For this review, take the finished solid that the model builds, in its own axes (mm). A direction names the side the tool comes from. Round coordinates to 2 decimals unless told otherwise and drop trailing zeros. Write each loop counter-clockwise with the first axis right and the second up, starting at its lowest first coordinate (ties: lowest second). Pieces come first, ordered by that corner, then holes. Notation, with made-up numbers: M 88.5,42 L 116.5,42 A13 ccw 116.5,67 Z; hole C 1,55.25 d10. An arc over 180 degrees is marked long. Use one line per item in the form item = value. Start each with the question number.
Item 1: Add section B-B (x = -4.5). State the section outline as (y, z) points.
Item 2: Add section C-C (y = 4.7). State the section outline as (x, z) points, and give its area (3 significant figures).
Item 3: For faces 1 (the flat face through (62.7, 3, -0.6)), 2 (the flat face through (19.94, 2.96, 59.46)), 3 (the flat face through (-40.765, 2.958, 53.771)), 4 (the flat face through (18.81, 2.96, -59.82)), list the 3-axis set-ups (+Z, -Z, +X, -X, +Y, -Y) from which the entire face can be reached by the end or side of a thin tool; tool diameter is ignored.
Item 4: For line 1 (X direction, y = 1.2, z = 0); line 2 (X direction, y = 1.3, z = -24); line 3 (Z direction, x = -42.5, y = 4.3), list the stretches that pass through material, from the lowest coordinate up. Write a range as [from, to].
Item 5: Add section A-A (z = -30). State the section outline as (x, y) points.
Item 6: Draft analysis for pull direction X (two halves, no side actions). For faces 5 (the cylindrical face through (-17.345, 2.958, 68.973)), 6 (the flat face through (64.59, 2.96, -19.54)), 7 (the cylindrical face through (54.57, 2.96, -45.61)), state which applies: released by +X, released by -X, zero draft, split by the parting line, or undercut.
Item 7: For P1, Ø3, axis at x = 5, y = 5, coming from the -Z side; P2, Ø1, axis at x = -9, y = 1, coming from the -Z side, all flat-tipped, find the tip position at first contact; note any pin that passes through.
Item 8: Add section D-D (z = 0). State the section outline as (x, y) points.
from build123d import *

# Parameters (mm, degrees)
SKETCH1_R           = 3.3
SKETCH1_R_2         = 50.8
BOSS_EXTRUDE1_DEPTH = 6


with BuildPart() as part:
    # Sketch1 → Boss-Extrude1 (new body)
    with BuildSketch(Plane(origin=(0, 0, 0), x_dir=(1, 0, 0), z_dir=(0, 1, 0))):
        with BuildLine():
            ThreePointArc((-50.084292244, 23.446975703), (-54.118923856, 17.647036419), (-60.96, 19.41260294))
            Line((-60.96, 19.41260294), (-66.591321273, 24.972992034))
            ThreePointArc((-66.591321273, 24.972992034), (-70.926140308, -5.247572863), (-62.191041695, -34.501141038))
            Line((-62.191041695, -34.501141038), (-38.242542673, -40.255931215))
            ThreePointArc((-38.242542673, -40.255931215), (-34.829443057, -42.441548483), (-33.501782647, -46.270842108))
            ThreePointArc((-33.501782647, -46.270842108), (-34.53819598, -49.698469864), (-37.300158502, -51.97758102))
            Line((-37.300158502, -51.97758102), (-44.328576757, -55.615031086))
            ThreePointArc((-44.328576757, -55.615031086), (-16.926644335, -69.07635711), (13.594446222, -69.808634365))
            Line((13.594446222, -69.808634365), (26.468070107, -48.810586278))
            ThreePointArc((26.468070107, -48.810586278), (33.175934652, -46.026293541), (37.90723426, -51.536514664))
            Line((37.90723426, -51.536514664), (39.194754164, -59.344971531))
            ThreePointArc((39.194754164, -59.344971531), (60.464898794, -37.44396365), (70.592871518, -8.642967708))
            Line((70.592871518, -8.642967708), (54.600709616, 10.089329884))
            ThreePointArc((54.600709616, 10.089329884), (54.025534005, 17.329281943), (60.728117694, 20.126263296))
            Line((60.728117694, 20.126263296), (68.552267011, 18.937821619))
            ThreePointArc((68.552267011, 18.937821619), (54.296006916, 45.9347149), (30.03434774, 64.466986558))
            Line((30.03434774, 64.466986558), (7.277024245, 55.04613507))
            ThreePointArc((7.277024245, 55.04613507), (0.213681623, 56.736378783), (-0.375193452, 63.975229447))
            Line((-0.375193452, 63.975229447), (3.172876855, 71.049188964))
            ThreePointArc((3.172876855, 71.049188964), (-26.908121067, 65.833178722), (-52.030623785, 48.485756553))
            Line((-52.030623785, 48.485756553), (-50.103261295, 23.931052539))
            ThreePointArc((-50.103261295, 23.931052539), (-50.089036326, 23.68919988), (-50.084292244, 23.446975703))
        make_face()
        with Locations(Location((-18.837675977, -57.976405233, 0), (0, 0, 270))):
            Circle(SKETCH1_R, mode=Mode.SUBTRACT)
        with Locations(Location((-60.96, 0, 0), (0, 0, 270))):
            Circle(SKETCH1_R, mode=Mode.SUBTRACT)
        with Locations(Location((49.317675977, -35.83138898, 0), (0, 0, 270))):
            Circle(SKETCH1_R, mode=Mode.SUBTRACT)
        with Locations(Location((-18.837675977, 57.976405233, 0), (0, 0, 270))):
            Circle(SKETCH1_R, mode=Mode.SUBTRACT)
        with Locations(Location((0, 0, 0), (0, 0, 270))):
            Circle(SKETCH1_R_2, mode=Mode.SUBTRACT)
        with Locations(Location((49.317675977, 35.83138898, 0), (0, 0, 270))):
            Circle(SKETCH1_R, mode=Mode.SUBTRACT)
    extrude(amount=BOSS_EXTRUDE1_DEPTH)


solid = part.part
Calculated:
q1.outline = M 0,-70.98 L 6,-70.98 L 6,-50.6 L 0,-50.6 Z; M 0,50.6 L 6,50.6 L 6,70.98 L 0,70.98 Z
q2.outline = M -66.59,-24.97 L -60.96,-19.41 A6.19 cw -50.1,-23.93 L -52.03,-48.49 A71.12 ccw 3.17,-71.05 L -0.38,-63.98 A6.19 cw 7.28,-55.05 L 30.03,-64.47 A71.12 ccw 68.55,-18.94 L 60.73,-20.13 A6.19 cw 54.6,-10.09 L 70.59,8.64 A71.12 ccw 39.19,59.34 L 37.91,51.54 A6.19 cw 26.47,48.81 L 13.59,69.81 A71.12 ccw -44.33,55.62 L -37.3,51.98 A6.19 cw -38.24,40.26 L -62.19,34.5 A71.12 ccw Z; hole C -60.96,0 d6.6; hole C 0,0 d101.6; hole C -18.84,-57.98 d6.6; hole C -18.84,57.98 d6.6; hole C 49.32,-35.83 d6.6; hole C 49.32,35.83 d6.6
q2.area = 6,080 mm^2
q3.face_1 = +X, +Y, -Y
q3.face_2 = +Z, +Y, -Y
q3.face_3 = -X, +Y, -Y
q3.face_4 = -Z, +Y, -Y
q4.line_1 = [-71.12, -64.26], [-57.66, -50.8], [50.8, 63.21]
q4.line_2 = [-66.95, -65.61], [-50.11, -44.77], [44.77, 66.95]
q4.line_3 = [-57.02, -27.83], [27.83, 39.23], [54.67, 57.02]
q5.outline = M -50.58,0 L -41,0 L -41,6 L -50.58,6 Z; M 41,0 L 64.48,0 L 64.48,6 L 41,6 Z
q6.face_5 = split by the parting line
q6.face_6 = undercut
q6.face_7 = released by +X
q7.P1 = -54.78
q7.P2 = -70.61
q8.outline = M -71.12,0 L -64.26,0 L -64.26,6 L -71.12,6 Z; M -57.66,0 L -50.8,0 L -50.8,6 L -57.66,6 Z; M 50.8,0 L 63.21,0 L 63.21,6 L 50.8,6 Z
